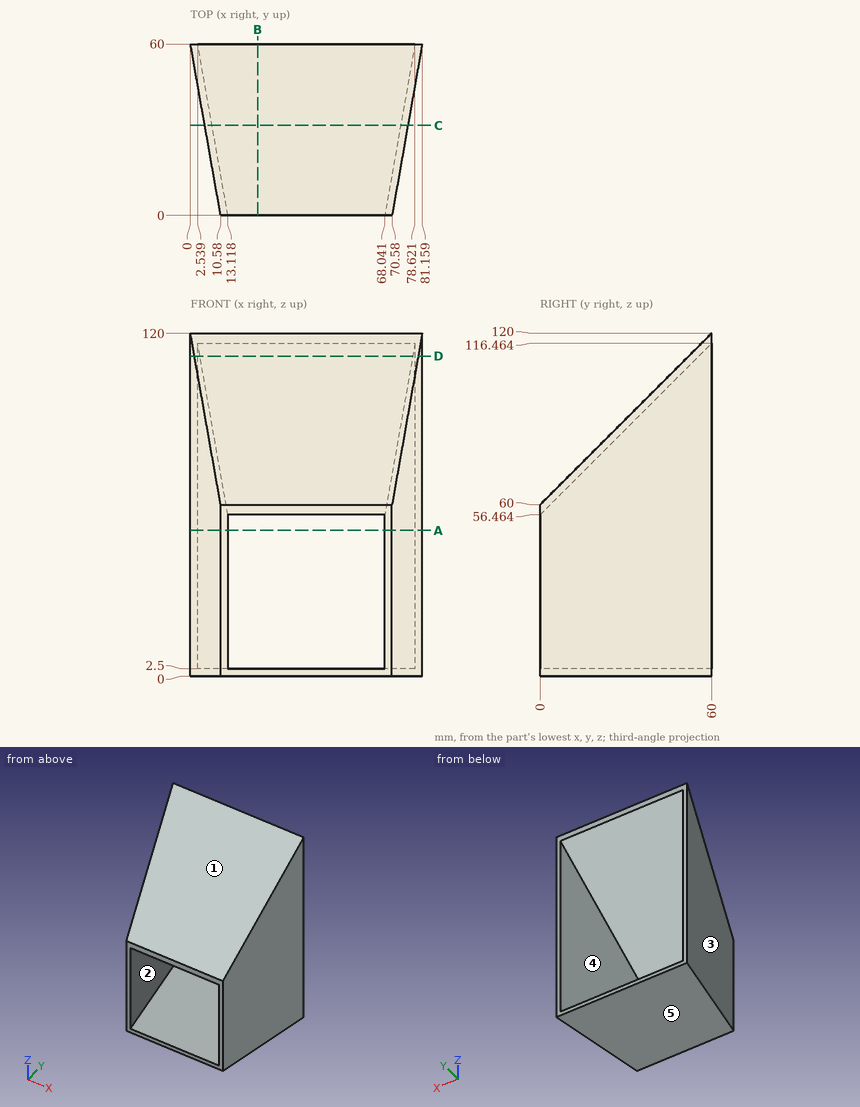
Geometry: see drawing. Coordinates: mm, zero at the bounding-box minimum. A direction names the side the tool comes from. Round coordinates to 2 decimals unless told otherwise and drop trailing zeros. Loops run counter-clockwise (first coordinate to the right, second up) from the corner with the lowest first, then second, coordinate; pieces in that order, holes last. Notation, with made-up numbers: (6.5, 81.25) -> (34.5, 81.25) arc R4 ccw to (34.5, 85.25) -> close; hole circle Ø6 at (18, 25). An arc over 180 degrees is marked (long way). Use one line per item in the form item = value. Start each with the question number.
Item 1: Section query D-D on z = 112. Return the cut outline in (x, y) (1 decimal), then the cut area to 3 significant figures.
Item 2: Section query B-B on x = 23.5. Return the cut outline in (y, z) (1 decimal), then the cut area to 3 significant figures.
Item 3: Section query C-C on y = 31.5. Return the cut outline in (x, z) (1 decimal).
Item 4: Section query A-A on z = 51. Return the cut outline in (x, y).
Item 5: Mould query, pull axis Z, two halves, no side actions, for the marked faces 1, 2 and 3. Classes: pulls with the +Z half, pulls with the -Z half, needs draft (parallel to the pull), parting line crosses it, or undercut.
Item 6: Material intervals for L1, parallel to X at y = 7, z = 21.5 (1 decimal); L2, parallel to X at y = 8.5, z = 41; L3, parallel to Z at x = 25, y = 31 (1 decimal), sorted ascending. Write a range as from..to.
Item 7: Contact query for flat-ended pins moving along their axis: pin 1 Ø12 at (y, z) = (10, 47.5) entering from +X; pin 2 Ø6 at (x, z) = (64.5, 94) entering from -Y; pin 3 Ø3 at (y, z) = (53, 66.5) entering from +X. Output: stop coordinate, or through.
Item 8: Set-up query: the marked faces 4 and 5. Return all of +Z, -Z, +X, -X, +Y, -Y with unobstructed straight access to the full face (end or side cutting, diameter ignored); none if empty.
Ans:
q1.outline = (0, 60) -> (1.4, 52) -> (79.7, 52) -> (81.2, 60) -> (78.6, 60) -> (77.8, 55.5) -> (3.3, 55.5) -> (2.5, 60) -> close
q1.area = 302 mm^2
q2.outline = (0, 0) -> (60, 0) -> (60, 2.5) -> (0, 2.5) -> close; (0, 56.5) -> (60, 116.5) -> (60, 120) -> (0, 60) -> close
q2.area = 362 mm^2
q3.outline = (5, 0) -> (76.1, 0) -> (76.1, 91.5) -> (5, 91.5) -> close; hole (7.6, 2.5) -> (73.6, 2.5) -> (73.6, 88) -> (7.6, 88) -> close
q4.outline = (0, 60) -> (10.58, 0) -> (13.12, 0) -> (2.54, 60) -> close; (68.04, 0) -> (70.58, 0) -> (81.16, 60) -> (78.62, 60) -> close
q5.face_1 = pulls with the +Z half
q5.face_2 = undercut
q5.face_3 = needs draft
q6.L1 = 9.3..11.9, 69.3..71.8
q6.L2 = 9.08..11.62, 69.54..72.08
q6.L3 = 0..2.5, 87.5..91
q7.pin_1 = 73.4
q7.pin_2 = 31
q7.pin_3 = 80.19
q8.face_4 = +Y
q8.face_5 = -Z, +X, -X, +Y, -Y
